Build history of the part. All positions in model axes, mm. A direction names the side the tool comes from. Give positions to 0.01 mm unless a question says otherwise; leave off trailing zeros. Order: outer loops, then holes, each group sorted by start corner. A loop starts at its lowest first (then second) coordinate and runs counter-clockwise, first axis right, second up. Notation, with made-up numbers: (65, -26.75) - (104, -26.75) arc R22 ccw to (104, -12.75) - close; hole circle Ø3 at (73, 8). An arc over 180 degrees is marked (long way). Answer in a Markdown table with one row per item.
```python
from build123d import *

# Parameters (mm, degrees)
SKICA1_W                 = 54.6
SKICA1_H                 = 54.6
P_IDAT_VYSUNUT_M2_DEPTH  = 3
SKICA4_W                 = 25
SKICA4_H                 = 5
ODEBRAT_VYSUNUT_M1_DEPTH = 2
SKICA5_W                 = 54.6
SKICA5_H                 = 5
ODEBRAT_VYSUNUT_M3_DEPTH = 1
SKICA14_W                = 52.6
SKICA14_H                = 1
P_IDAT_VYSUNUT_M9_DEPTH  = 9.5
SKICA17_R                = 2
ODEBRAT_VYSUNUT_M8_DEPTH = 4
SKICA19_W                = 6.8
SKICA19_H                = 6.8
P_IDAT_VYSUNUT_M10_DEPTH = 12.5
SKICA20_R                = 2.4
ODEBRAT_VYSUNUT_M9_DEPTH = 1.7
ZAOBLIT1_R               = 2.5


with BuildPart() as part:
    # Skica1 → Přidat vysunutím2 (new body)
    with BuildSketch(Plane.XY):
        Rectangle(SKICA1_W, SKICA1_H)
    extrude(amount=P_IDAT_VYSUNUT_M2_DEPTH)

    # Skica4 → Odebrat vysunutím1 (cut)
    with BuildSketch(Plane.XY.offset(3)):
        Rectangle(SKICA4_W, SKICA4_H)
    extrude(amount=-ODEBRAT_VYSUNUT_M1_DEPTH, mode=Mode.SUBTRACT)

    # Skica5 → Odebrat vysunutím3 (cut)
    with BuildSketch(Plane(origin=(0, 0, 0), x_dir=(-1, 0, 0), z_dir=(0, 0, -1))):
        Rectangle(SKICA5_W, SKICA5_H)
    extrude(amount=-ODEBRAT_VYSUNUT_M3_DEPTH, mode=Mode.SUBTRACT)

    # Skica14 → Přidat vysunutím9 (add)
    with BuildSketch(Plane.XY.offset(3)):
        Polygon((27.3, 27.3), (-27.3, 27.3), (-27.3, -27.3), (-26.3, -27.3), (-26.3, -26.3), (-26.3, 26.3), (26.3, 26.3), (26.3, -26.3), (26.3, -27.3), (27.3, -27.3), align=None)
        with Locations((0, -26.8)):
            Rectangle(SKICA14_W, SKICA14_H)
    extrude(amount=P_IDAT_VYSUNUT_M9_DEPTH)

    # Skica17 → Odebrat vysunutím8 (cut)
    with BuildSketch(Plane(origin=(0, 0, 1), x_dir=(-1, 0, 0), z_dir=(0, 0, -1))):
        with Locations((-20.3, 0)):
            Circle(SKICA17_R)
        with Locations((20.3, 0)):
            Circle(SKICA17_R)
    extrude(amount=-ODEBRAT_VYSUNUT_M8_DEPTH, mode=Mode.SUBTRACT)

    # Skica19 → Přidat vysunutím10 (add)
    with BuildSketch(Plane(origin=(0, 0, 0), x_dir=(-1, 0, 0), z_dir=(0, 0, -1))):
        with Locations((-23.9, 23.9)):
            Rectangle(SKICA19_W, SKICA19_H)
        with Locations((23.9, 23.9)):
            Rectangle(SKICA19_W, SKICA19_H)
        with Locations((-23.9, -23.9)):
            Rectangle(SKICA19_W, SKICA19_H)
        with Locations((23.9, -23.9)):
            Rectangle(SKICA19_W, SKICA19_H)
    extrude(amount=-P_IDAT_VYSUNUT_M10_DEPTH)

    # Skica20 → Odebrat vysunutím9 (cut)
    with BuildSketch(Plane.XY.offset(12.5)):
        with Locations((-23.4, -23.4)):
            Circle(SKICA20_R)
        with Locations((-23.4, 23.4)):
            Circle(SKICA20_R)
        with Locations((23.400280565, 23.4)):
            Circle(SKICA20_R)
        with Locations((23.400280565, -23.4)):
            Circle(SKICA20_R)
    extrude(amount=-ODEBRAT_VYSUNUT_M9_DEPTH, mode=Mode.SUBTRACT)

    # Zaoblit1
    zaoblit1_edges = [part.edges().sort_by_distance(p)[0] for p in [
        (-20.5, 20.5, 7.75),
        (20.5, -20.5, 7.75),
        (-20.5, -20.5, 7.75),
        (20.5, 20.5, 7.75),
    ]]
    fillet(zaoblit1_edges, radius=ZAOBLIT1_R)


solid = part.part
```
1. Cut at C-C on y = 0. Write the cut outline in (x, z).
Check result:
| item | result |
|---|---|
| outline | (-27.3, 1) - (-22.3, 1) - (-22.3, 3) - (-26.3, 3) - (-26.3, 12.5) - (-27.3, 12.5) - close; (-18.3, 1) - (-12.5, 1) - (-12.5, 3) - (-18.3, 3) - close; (12.5, 1) - (18.3, 1) - (18.3, 3) - (12.5, 3) - close; (22.3, 1) - (27.3, 1) - (27.3, 12.5) - (26.3, 12.5) - (26.3, 3) - (22.3, 3) - close |
2. Two-plate mould, pull along Y, no slides. Class faces 5 (the face through (0, 26.3, 8)), 6 (the face through (0, 27.3, 6)), 7 (the face through (0, -15, 0)): +Y half, -Y half, draft (parallel to the pull), parting line (faces both ways), or undercut.
Check result:
| item | result |
|---|---|
| face 5 | undercut |
| face 6 | +Y half |
| face 7 | draft |
3. Cut at D-D on y = 9.5. Write the cut outline in (x, z), and give its area (3 significant figures).
Check result:
| item | result |
|---|---|
| outline | (-27.3, 0) - (27.3, 0) - (27.3, 12.5) - (26.3, 12.5) - (26.3, 3) - (-26.3, 3) - (-26.3, 12.5) - (-27.3, 12.5) - close |
| area | 183 mm² |
4. Which spindle directions (+Z, -Z, +X, -X, +Y, -Y) get a long thin tool onto all of the face, cutting with end or side? Do faces 1 (the face through (12.5, 0, 2)), 2 (the face through (-27.3, 0, 6)), 3 (the face through (0, 2.5, 1)), 4 (the face through (26.3, 0, 8)). Say none if no direction does.
Check result:
| item | result |
|---|---|
| face 1 | +Z, -Z |
| face 2 | +Z, -Z, -X, +Y, -Y |
| face 3 | -Z |
| face 4 | +Z |
5. Cut at B-B on z = 9.25. Write the cut outline in (x, y).
Check result:
| item | result |
|---|---|
| outline | (-27.3, -27.3) - (27.3, -27.3) - (27.3, 27.3) - (-27.3, 27.3) - close; hole (-26.3, -20.5) - (-23, -20.5) arc R2.5 cw to (-20.5, -23) - (-20.5, -26.3) - (20.5, -26.3) - (20.5, -23) arc R2.5 cw to (23, -20.5) - (26.3, -20.5) - (26.3, 20.5) - (23, 20.5) arc R2.5 cw to (20.5, 23) - (20.5, 26.3) - (-20.5, 26.3) - (-20.5, 23) arc R2.5 cw to (-23, 20.5) - (-26.3, 20.5) - close |
6. Probe line 1 (Y direction, x = -23.4, z = 12.2); line 2 (Y direction, x = 20.3, z = 1.65); line 3 (X direction, y = -12, z = 4.5). List the from-to ranges inside material, lowest first.
Check result:
| item | result |
|---|---|
| line 1 | y = -27.3 to -25.8, -21 to -20.5, 20.5 to 21, 25.8 to 27.3 |
| line 2 | y = -27.3 to -2, 2 to 27.3 |
| line 3 | x = -27.3 to -26.3, 26.3 to 27.3 |
7. Cut at A-A on x = 1.5. Write the cut outline in (y, z), and give its area (3 significant figures).
Check result:
| item | result |
|---|---|
| outline | (-27.3, 0) - (-2.5, 0) - (-2.5, 3) - (-26.3, 3) - (-26.3, 12.5) - (-27.3, 12.5) - close; (2.5, 0) - (27.3, 0) - (27.3, 12.5) - (26.3, 12.5) - (26.3, 3) - (2.5, 3) - close |
| area | 168 mm² |
8. Drop flat-ended pins along their axis: P1, Ø8, axis at x = 15, y = 9, coming from the +Z side; P2, Ø4, axis at x = -23.5, y = -23.5, coming from the +Z side. Give the stop position or say it passes through.
Check result:
| item | result |
|---|---|
| P1 | stops at z = 3 |
| P2 | stops at z = 10.8 |
